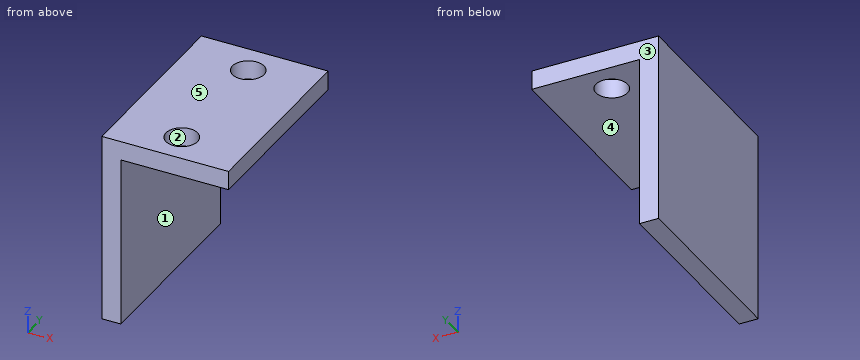
```python
from build123d import *

# Parameters (mm, degrees)
BOSS_EXTRUDE1_DEPTH = 30
SKETCH2_R           = 2.5
CUT_EXTRUDE1_DEPTH  = 31


with BuildPart() as part:
    # Sketch1 → Boss-Extrude1 (new body)
    with BuildSketch(Plane(origin=(0, 0, 0), x_dir=(1, 0, 0), z_dir=(0, 1, 0))):
        Polygon((0, 30), (0, 0), (20, 0), (20, 3), (3, 3), (3, 30), align=None)
    extrude(amount=BOSS_EXTRUDE1_DEPTH)

    # Sketch2 → Cut-Extrude1 (cut, through all)
    with BuildSketch(Plane.XY):
        with Locations((10, 25)):
            Circle(SKETCH2_R)
        with Locations((10, 5)):
            Circle(SKETCH2_R)
    extrude(amount=-CUT_EXTRUDE1_DEPTH, mode=Mode.SUBTRACT)


solid = part.part
```
Geometry check sheet. Reference: the model listing, model coordinates, mm. Face numbers are marked on the shaded views. A direction names the side the tool comes from. Round coordinates to 2 decimals unless told otherwise and drop trailing zeros. Loops run counter-clockwise (first coordinate to the right, second up) from the corner with the lowest first, then second, coordinate; pieces in that order, holes last. Notation, with made-up numbers: M 40,81.5 L 95,81.5 A22 ccw 95,118.5 Z; hole C 55.5,4 d1. An arc over 180 degrees is marked long. Return JSON: item names as keys, results as strings. Group by question number.
(1) Section check A-A, the plane x = 10. Enter the section's corners in (y, z).
(2) Section check C-C, the plane y = 16.5. Enter the section's corners in (x, z), and give its area (3 significant figures).
(3) Mould release check, pull along Y, two halves, no side actions. Record for the marked faces 1, 2 and 3: pulls with the +Y half, pulls with the -Y half, needs draft (parallel to the pull), parting line crosses it, or undercut.
(4) Go/stop test with flat-tipped pins: pin 1 (10 mm diameter, centred on x = 8, y = 7.5, fed in from +Z); pin 2 (6 mm diameter, centred on y = 14, z = -22.5, fed in from +X); pin 3 (4 mm diameter, centred on x = 11, y = 3.5, fed in from -Z). Record where each tip stops, or that it passes through.
(5) Section check B-B, the plane y = 25. Enter the section's corners in (x, z).
(6) Set-up check for the marked faces 4 and 5: record each of +Z, -Z, +X, -X, +Y, -Y from which the full face is reachable in a straight line by a thin tool's end or side.
(7) Section check D-D, the plane z = -22. Enter the section's corners in (x, y), and give its area (3 significant figures).
(8) Scan lines: line 1 along Y through (x, z) = (10, -1.1); line 2 along Z through (x, y) = (9.75, 28.5); line 3 along X through (y, z) = (9.75, -25). Record each from-to range of solid material in increasing order. Write a range as [from, to].
Data:
{
 "1": {"outline": "M 0,-3 L 2.5,-3 L 2.5,0 L 0,0 Z; M 7.5,-3 L 22.5,-3 L 22.5,0 L 7.5,0 Z; M 27.5,-3 L 30,-3 L 30,0 L 27.5,0 Z"},
 "2": {"outline": "M 0,-30 L 3,-30 L 3,-3 L 20,-3 L 20,0 L 0,0 Z", "area": "141 mm²"},
 "3": {"face 1": "needs draft", "face 2": "undercut", "face 3": "pulls with the +Y half"},
 "4": {"pin 1": "z = 0", "pin 2": "x = 3", "pin 3": "z = -3"},
 "5": {"outline": "M 0,-30 L 3,-30 L 3,-3 L 7.5,-3 L 7.5,0 L 0,0 Z; M 12.5,-3 L 20,-3 L 20,0 L 12.5,0 Z"},
 "6": {"face 4": "-Z, +X, +Y, -Y", "face 5": "+Z, +X, -X, +Y, -Y"},
 "7": {"outline": "M 0,0 L 3,0 L 3,30 L 0,30 Z", "area": "90.0 mm²"},
 "8": {"line 1": "[0, 2.5], [7.5, 22.5], [27.5, 30]", "line 2": "[-3, 0]", "line 3": "[0, 3]"}
}
